For this review, take the finished solid that the model builds, in its own axes (mm). A direction names the side the tool comes from. Round coordinates to 2 decimals unless told otherwise and drop trailing zeros. Order: outer loops, then holes, each group sorted by start corner. A loop starts at its lowest first (then second) coordinate and runs counter-clockwise, first axis right, second up. Notation, with made-up numbers: (45.25, -18) -> (95.25, -18) arc R19 ccw to (95.25, -12) -> close; hole circle Ø8 at (81.25, 80). An arc over 180 degrees is marked (long way). Put each result on its own line as item: value. Start each with the question number.
```python
from build123d import *

# Parameters (mm, degrees)
SKETCH1_W               = 128
SKETCH1_H               = 41
BOSS_EXTRUDE1_DEPTH     = 3
CUT_EXTRUDE2_START      = -4
CUT_EXTRUDE2_DEPTH      = 5
LPATTERN3_COUNT         = 12
LPATTERN3_PITCH         = 10
CUT_EXTRUDE3_START      = -4
CUT_EXTRUDE3_DEPTH      = 5
LPATTERN5_COUNT         = 12
LPATTERN5_PITCH         = 10
CUT_EXTRUDE4_START      = -4
SKETCH6_R               = 1.6
CUT_EXTRUDE4_DEPTH      = 5
MIRROR3_START           = -4
MIRROR3_COPY_1_SKETCH_R = 1.6
MIRROR3_COPY_1_DEPTH    = 5
CUT_EXTRUDE5_START      = -4
CUT_EXTRUDE5_DEPTH      = 5
CUT_EXTRUDE6_START      = -4
SKETCH8_W               = 4
SKETCH8_H               = 5
CUT_EXTRUDE6_DEPTH      = 5


with BuildPart() as part:
    # Sketch1 → Boss-Extrude1 (new body)
    with BuildSketch(Plane(origin=(0, 0, 0), x_dir=(1, 0, 0), z_dir=(0, 1, 0))):
        Rectangle(SKETCH1_W, SKETCH1_H)
    extrude(amount=BOSS_EXTRUDE1_DEPTH)

    # Sketch2 → Cut-Extrude2 (cut)
    with BuildSketch(Plane(origin=(0, 3, 0), x_dir=(1, 0, 0), z_dir=(0, 1, 0)).offset(CUT_EXTRUDE2_START)):
        Polygon((-60, 20.5), (-55, 15.5), (-50, 20.5), align=None)
    cut_extrude2 = extrude(amount=CUT_EXTRUDE2_DEPTH, mode=Mode.SUBTRACT)

    # LPattern3: Cut-Extrude2 ×12
    with Locations(*[(i * LPATTERN3_PITCH, 0, 0) for i in range(1, LPATTERN3_COUNT)]):
        add(cut_extrude2, mode=Mode.SUBTRACT)

    # Sketch5 → Cut-Extrude3 (cut)
    with BuildSketch(Plane(origin=(0, 3, 0), x_dir=(1, 0, 0), z_dir=(0, 1, 0)).offset(CUT_EXTRUDE3_START)):
        Polygon((-55, -20.5), (-60, -15.5), (-60, -20.5), align=None)
        Polygon((-50, -15.5), (-55, -20.5), (-50, -20.5), align=None)
    cut_extrude3 = extrude(amount=CUT_EXTRUDE3_DEPTH, mode=Mode.SUBTRACT)

    # LPattern5: Cut-Extrude3 ×12
    with Locations(*[(i * LPATTERN5_PITCH, 0, 0) for i in range(1, LPATTERN5_COUNT)]):
        add(cut_extrude3, mode=Mode.SUBTRACT)

    # Sketch6 → Cut-Extrude4 (cut)
    with BuildSketch(Plane(origin=(0, 3, 0), x_dir=(1, 0, 0), z_dir=(0, 1, 0)).offset(CUT_EXTRUDE4_START)):
        with Locations((-58.5, 4.5)):
            Circle(SKETCH6_R)
    cut_extrude4 = extrude(amount=CUT_EXTRUDE4_DEPTH, mode=Mode.SUBTRACT)

    # Mirror2: Cut-Extrude4 across plane
    add(cut_extrude4.mirror(Plane(origin=(0, 0, 0), x_dir=(0, 0, 1), z_dir=(1, 0, 0))), mode=Mode.SUBTRACT)

    # Mirror3: Cut-Extrude4 across plane
    add(cut_extrude4.mirror(Plane.XY), mode=Mode.SUBTRACT)

    # Mirror3 copy 1 sketch → Mirror3 copy 1 (cut)
    with BuildSketch(Plane(origin=(0, 3, 0), x_dir=(-1, 0, 0), z_dir=(0, 1, 0)).offset(MIRROR3_START)):
        with Locations((-58.5, 4.5)):
            Circle(MIRROR3_COPY_1_SKETCH_R)
    extrude(amount=MIRROR3_COPY_1_DEPTH, mode=Mode.SUBTRACT)

    # Sketch7 → Cut-Extrude5 (cut)
    with BuildSketch(Plane(origin=(0, 3, 0), x_dir=(1, 0, 0), z_dir=(0, 1, 0)).offset(CUT_EXTRUDE5_START)):
        Polygon((-60, 20.5), (-64, 10.5), (-64, 20.5), align=None)
    cut_extrude5 = extrude(amount=CUT_EXTRUDE5_DEPTH, mode=Mode.SUBTRACT)

    # Mirror4: Cut-Extrude5 across plane
    add(cut_extrude5.mirror(Plane(origin=(0, 0, 0), x_dir=(0, 0, 1), z_dir=(1, 0, 0))), mode=Mode.SUBTRACT)

    # Sketch8 → Cut-Extrude6 (cut)
    with BuildSketch(Plane(origin=(0, 3, 0), x_dir=(1, 0, 0), z_dir=(0, 1, 0)).offset(CUT_EXTRUDE6_START)):
        with Locations((-62, -18)):
            Rectangle(SKETCH8_W, SKETCH8_H)
    cut_extrude6 = extrude(amount=CUT_EXTRUDE6_DEPTH, mode=Mode.SUBTRACT)

    # Mirror5: Cut-Extrude6 across plane
    add(cut_extrude6.mirror(Plane(origin=(0, 0, 0), x_dir=(0, 0, 1), z_dir=(1, 0, 0))), mode=Mode.SUBTRACT)


solid = part.part
```
Item 1: Insertion check: pin 1 Ø1.9 at (x, z) = (58.5, 4.5) entering from +Y; pin 2 Ø1 at (x, y) = (33.5, 1.5) entering from +Z. Each pin has a flat end and moves straight along its axis. Give the tip position at first contact, or say it passes through.
Item 2: Consider section B-B, the plane x = -58.5. Write out the cut boundary in (y, z).
Item 3: Consider section C-C, the plane y = 1.45. Count the separate pieces of the cut face and the enclosed holes in it, plus the area to 3 significant figures.
Item 4: For L1, parallel to X at y = 0.5, z = -5; L2, parallel to Z at x = 58.5, y = 0.9; L3, parallel to Z at x = 39.5, y = 1.05, list the stretches that pass through material, from the lowest coordinate up.
Item 5: Mouldability with a two-part tool opening along X and no side actions: class faces 1 (the face through (56.974, 1.479, -4.981)), 2 (the face through (61.97, 1.48, -15.57)), 3 (the face through (27.5, 1.5, -18)), 4 (the face through (-1, 0, 0)) as +X half, -X half, draft (parallel to the pull), parting line (faces both ways), or undercut.
Item 6: Consider section D-D, the plane x = 18.5. Write out the cut boundary in (y, z).
Item 7: Tool access review of faces 5 (the face through (-42.5, 1.5, -18)), 6 (the face through (7.5, 1.5, 18)): name each direction out of +Z, -Z, +X, -X, +Y, -Y from which nothing blocks a thin tool from reaching the whole face with its end or side.
Item 8: Consider section A-A, the plane z = 4.5. Write out the cut boundary in (x, y).
Evaluation:
1. pin 1: passes through
1. pin 2: stops at z = 19.5
2. outline: (0, -19) -> (3, -19) -> (3, -6.1) -> (0, -6.1) -> close; (0, -2.9) -> (3, -2.9) -> (3, 2.9) -> (0, 2.9) -> close; (0, 6.1) -> (3, 6.1) -> (3, 17) -> (0, 17) -> close
3. separate pieces: 1
3. enclosed holes: 4
3. area: 4,540 mm^2
4. L1: x = -64 to -60.02, -56.98 to 56.98, 60.02 to 64
4. L2: z = -19 to -6.1, -2.9 to 2.9, 6.1 to 17
4. L3: z = -20 to 16
5. face 1: undercut
5. face 2: +X half
5. face 3: undercut
5. face 4: draft
6. outline: (0, -19) -> (3, -19) -> (3, 17) -> (0, 17) -> close
7. face 5: -Z, +Y, -Y
7. face 6: +Z, +Y, -Y
8. outline: (-64, 0) -> (-60.1, 0) -> (-60.1, 3) -> (-64, 3) -> close; (-56.9, 0) -> (56.9, 0) -> (56.9, 3) -> (-56.9, 3) -> close; (60.1, 0) -> (64, 0) -> (64, 3) -> (60.1, 3) -> close
